Design review of the part built by this model. Coordinates are the model's own, in mm. A direction names the side the tool comes from. Give positions to 0.01 mm unless a question says otherwise; leave off trailing zeros. Order: outer loops, then holes, each group sorted by start corner. A loop starts at its lowest first (then second) coordinate and runs counter-clockwise, first axis right, second up. Notation, with made-up numbers: (54.5, 6) -> (85.5, 6) arc R17 ccw to (85.5, 19) -> close; hole circle Ø6 at (16, -30.75). An arc over 180 degrees is marked (long way). Return JSON: item names as keys, results as strings.
```python
from build123d import *

# Parameters (mm, degrees)
SKETCH1_W               = 80
SKETCH1_H               = 40
SKETCH1_R               = 2.25
BOSS_EXTRUDE1_DEPTH     = 5
BOSS_EXTRUDE1_2_DEPTH   = 5
SKETCH2_W               = 80
SKETCH2_H               = 5
BOSS_EXTRUDE2_DEPTH     = 71.3
SKETCH3_W               = 43.85
SKETCH3_H               = 62
BOSS_EXTRUDE3_DEPTH     = 5
SKETCH5_W               = 29.85
SKETCH5_H               = 38
CUT_EXTRUDE2_DEPTH      = 10
CUT_EXTRUDE1_REACH      = 114.097
SKETCH4_R               = 1.3
FILLET1_R               = 3
FILLET2_R               = 3
CUT_EXTRUDE3_DEPTH      = 133.735413511
CUT_EXTRUDE3_DEPTH_BACK = 133.735413511
SKETCH6_W               = 50
SKETCH6_H               = 38.3
FILLET3_R               = 3
SKETCH9_R               = 2.65
SKETCH9_R_2             = 1.05
BOSS_EXTRUDE5_DEPTH     = 4.75
SKETCH10_W              = 12
SKETCH10_H              = 6.8
CUT_EXTRUDE4_DEPTH      = 8


with BuildPart() as part:
    # Sketch1 → Boss-Extrude1 (new body)
    with BuildSketch(Plane(origin=(0, 0, 0), x_dir=(1, 0, 0), z_dir=(0, 1, 0))):
        with Locations((0, 46)):
            Rectangle(SKETCH1_W, SKETCH1_H)
        with Locations(Location((-30.625, 53.044055982, 0), (0, 0, 270))):
            Circle(SKETCH1_R, mode=Mode.SUBTRACT)
        with Locations(Location((30.625, 53.044055982, 0), (0, 0, 90))):
            Circle(SKETCH1_R, mode=Mode.SUBTRACT)
    extrude(amount=BOSS_EXTRUDE1_DEPTH)



with BuildPart() as body_2:
    # Sketch1 → Boss-Extrude1 2 (new body)
    with BuildSketch(Plane(origin=(0, 0, 0), x_dir=(1, 0, 0), z_dir=(0, 1, 0))):
        with Locations((0, -46)):
            Rectangle(SKETCH1_W, SKETCH1_H)
        with Locations(Location((30.625, -53.044055982, 0), (0, 0, 270))):
            Circle(SKETCH1_R, mode=Mode.SUBTRACT)
        with Locations(Location((-30.625, -53.044055982, 0), (0, 0, 90))):
            Circle(SKETCH1_R, mode=Mode.SUBTRACT)
    extrude(amount=BOSS_EXTRUDE1_2_DEPTH)


with BuildPart() as part_1:
    add(part.part)

    add(body_2.part)  # Boss-Extrude2 merges body 2
    # Sketch2 → Boss-Extrude2 (add)
    with BuildSketch(Plane(origin=(0, 5, 0), x_dir=(1, 0, 0), z_dir=(0, 1, 0))):
        with Locations((0, 28.5)):
            Rectangle(SKETCH2_W, SKETCH2_H)
        with Locations((0, -28.5)):
            Rectangle(SKETCH2_W, SKETCH2_H)
    extrude(amount=BOSS_EXTRUDE2_DEPTH)

    # Sketch3 → Boss-Extrude3 (add)
    with BuildSketch(Plane(origin=(0, 76.3, 0), x_dir=(1, 0, 0), z_dir=(0, 1, 0))):
        with Locations((-3.925, 0)):
            Rectangle(SKETCH3_W, SKETCH3_H)
    extrude(amount=BOSS_EXTRUDE3_DEPTH)

    # Sketch5 → Cut-Extrude2 (cut)
    with BuildSketch(Plane.XZ.offset(-76.3)):
        with Locations((-3.925, 0)):
            Rectangle(SKETCH5_W, SKETCH5_H)
    extrude(amount=-CUT_EXTRUDE2_DEPTH, mode=Mode.SUBTRACT)

    # Sketch4 → Cut-Extrude1 (cut, up to next)
    with BuildSketch(Plane(origin=(0, 81.3, 0), x_dir=(1, 0, 0), z_dir=(0, 1, 0)), mode=Mode.PRIVATE) as cut_extrude1_sk1:
        with Locations(Location((-23, 20, 0), (0, 0, 270))):
            Circle(SKETCH4_R)
    cut_extrude1_tool1 = extrude(cut_extrude1_sk1.sketch, amount=-CUT_EXTRUDE1_REACH, mode=Mode.PRIVATE) & part_1.part
    # Sketch4 → Cut-Extrude1 (cut, up to next)
    with BuildSketch(Plane(origin=(0, 81.3, 0), x_dir=(1, 0, 0), z_dir=(0, 1, 0)), mode=Mode.PRIVATE) as cut_extrude1_sk2:
        with Locations(Location((15, 20, 0), (0, 0, 270))):
            Circle(SKETCH4_R)
    cut_extrude1_tool2 = extrude(cut_extrude1_sk2.sketch, amount=-CUT_EXTRUDE1_REACH, mode=Mode.PRIVATE) & part_1.part
    # Sketch4 → Cut-Extrude1 (cut, up to next)
    with BuildSketch(Plane(origin=(0, 81.3, 0), x_dir=(1, 0, 0), z_dir=(0, 1, 0)), mode=Mode.PRIVATE) as cut_extrude1_sk3:
        with Locations(Location((15, -20, 0), (0, 0, 270))):
            Circle(SKETCH4_R)
    cut_extrude1_tool3 = extrude(cut_extrude1_sk3.sketch, amount=-CUT_EXTRUDE1_REACH, mode=Mode.PRIVATE) & part_1.part
    # Sketch4 → Cut-Extrude1 (cut, up to next)
    with BuildSketch(Plane(origin=(0, 81.3, 0), x_dir=(1, 0, 0), z_dir=(0, 1, 0)), mode=Mode.PRIVATE) as cut_extrude1_sk4:
        with Locations(Location((-23, -20, 0), (0, 0, 270))):
            Circle(SKETCH4_R)
    cut_extrude1_tool4 = extrude(cut_extrude1_sk4.sketch, amount=-CUT_EXTRUDE1_REACH, mode=Mode.PRIVATE) & part_1.part
    add(cut_extrude1_tool1.solids().sort_by_distance((-23, 81.3, -20))[0], mode=Mode.SUBTRACT)
    add(cut_extrude1_tool2.solids().sort_by_distance((15, 81.3, -20))[0], mode=Mode.SUBTRACT)
    add(cut_extrude1_tool3.solids().sort_by_distance((15, 81.3, 20))[0], mode=Mode.SUBTRACT)
    add(cut_extrude1_tool4.solids().sort_by_distance((-23, 81.3, 20))[0], mode=Mode.SUBTRACT)

    # Fillet1
    fillet1_edges = [part_1.edges().sort_by_distance(p)[0] for p in [
        (0, 5, -31),
        (-3.925, 76.3, -26),
        (-3.925, 76.3, 26),
        (0, 5, 31),
    ]]
    fillet(fillet1_edges, radius=FILLET1_R)

    # Fillet2
    fillet2_edges = [part_1.edges().sort_by_distance(p)[0] for p in [
        (18, 76.3, -28.5),
        (-25.85, 76.3, -28.5),
        (-25.85, 76.3, 28.5),
        (18, 76.3, 28.5),
    ]]
    fillet(fillet2_edges, radius=FILLET2_R)

    # Sketch6 → Cut-Extrude3 (cut, two sides: drawn at the far end of the back side and taken through both)
    with BuildSketch(Plane.XY.offset(31).offset(-CUT_EXTRUDE3_DEPTH_BACK)):
        with Locations((0, 42.15)):
            Rectangle(SKETCH6_W, SKETCH6_H)
    extrude(amount=CUT_EXTRUDE3_DEPTH + CUT_EXTRUDE3_DEPTH_BACK, mode=Mode.SUBTRACT)

    # Fillet3
    fillet3_edges = [part_1.edges().sort_by_distance(p)[0] for p in [
        (-25, 61.3, -28.5),
        (-25, 61.3, 28.5),
        (-25, 23, -28.5),
        (-25, 23, 28.5),
        (25, 23, -28.5),
        (25, 23, 28.5),
        (25, 61.3, -28.5),
        (25, 61.3, 28.5),
        (-18.85, 78.8, -19),
        (-18.85, 78.8, 19),
        (11, 78.8, 19),
        (11, 78.8, -19),
    ]]
    fillet(fillet3_edges, radius=FILLET3_R)

    # Sketch9 → Boss-Extrude5 (add)
    # profile 1 of 4: a face of its own
    with BuildSketch(Plane.XZ.offset(-76.3)):
        with Locations(Location((-23, 20, 0), (0, 0, 270))):
            Circle(SKETCH9_R)
        with Locations(Location((-23, 20, 0), (0, 0, 270))):
            Circle(SKETCH9_R_2, mode=Mode.SUBTRACT)
    # profile 2 of 4: a face of its own
    with BuildSketch(Plane.XZ.offset(-76.3)):
        with Locations(Location((-23, -20, 0), (0, 0, 270))):
            Circle(SKETCH9_R)
        with Locations(Location((-23, -20, 0), (0, 0, 270))):
            Circle(SKETCH9_R_2, mode=Mode.SUBTRACT)
    # profile 3 of 4: a face of its own
    with BuildSketch(Plane.XZ.offset(-76.3)):
        with Locations(Location((15, 20, 0), (0, 0, 270))):
            Circle(SKETCH9_R)
        with Locations(Location((15, 20, 0), (0, 0, 270))):
            Circle(SKETCH9_R_2, mode=Mode.SUBTRACT)
    # profile 4 of 4: a face of its own
    with BuildSketch(Plane.XZ.offset(-76.3)):
        with Locations(Location((15, -20, 0), (0, 0, 270))):
            Circle(SKETCH9_R)
        with Locations(Location((15, -20, 0), (0, 0, 270))):
            Circle(SKETCH9_R_2, mode=Mode.SUBTRACT)
    extrude(amount=BOSS_EXTRUDE5_DEPTH)

    # Sketch10 → Cut-Extrude4 (cut)
    with BuildSketch(Plane.XY.offset(31)):
        with Locations((6.7, 73.45)):
            Rectangle(SKETCH10_W, SKETCH10_H)
    extrude(amount=-CUT_EXTRUDE4_DEPTH, mode=Mode.SUBTRACT)


solid = part_1.part
```
Item 1: Mouldability with a two-part tool opening along X and no side actions: class faces 1 (the face through (18.86, 77.2, 28.46)), 2 (the face through (10.1, 78.83, 18.14)), 3 (the face through (-1, 5, 50)) as released by +X, released by -X, zero draft, split by the parting line, or undercut.
Result set:
{"face 1": "released by +X", "face 2": "undercut", "face 3": "zero draft"}
Item 2: Add section D-D (y = 24.5). Give the boundary of the cut face in (x, z).
Result set:
{"outline": "(-40, -31) -> (-24.6, -31) -> (-24.6, -26) -> (-40, -26) -> close; (-40, 26) -> (-24.6, 26) -> (-24.6, 31) -> (-40, 31) -> close; (24.6, -31) -> (40, -31) -> (40, -26) -> (24.6, -26) -> close; (24.6, 26) -> (40, 26) -> (40, 31) -> (24.6, 31) -> close"}
Item 3: Wall thickness on L1, parallel to X at y = 79.05, z = -20; L2, parallel to Z at x = -3.5, y = 71; L3, parallel to Y at x = -15.5, z = 30.5: over which ranges is each line inside the solid? List them lowest first. Write a range as [from, to].
Result set:
{"L1": "x = [-25.85, -24.3], [-21.7, 13.7], [16.3, 18]", "L2": "z = [-31, -26], [26, 31]", "L3": "y = [0, 23], [61.3, 81.3]"}
Item 4: Machinability: for faces 4 (the face through (-4, 79, -19)), 5 (the face through (0, 61.3, 28)), 6 (the face through (-1, 5, -50)), 7 (the face through (7, 70.05, 29)), 8 (the face through (-24, 71.55, 19)), which of the approach directions +Z, -Z, +X, -X, +Y, -Y give a long, thin tool a straight path to every point of the face, cutting with its end or side? Answer none if there is none.
Result set:
{"face 4": "+Y, -Y", "face 5": "+Z, -Z", "face 6": "-Z, +X, -X, +Y", "face 7": "+Z", "face 8": "+X, -X, -Y"}
Item 5: Add section A-A (x = 2.5). Give the number of separate pieces and of enclosed holes in the cut face, plus the area to 3 significant figures.
Result set:
{"separate pieces": "5", "enclosed holes": "0", "area": "820 mm^2"}
Item 6: Add section C-C (y = 35). Give the boundary of the cut face in (x, z), plus the area to 3 significant figures.
Result set:
{"outline": "(-40, -31) -> (-25, -31) -> (-25, -26) -> (-40, -26) -> close; (-40, 26) -> (-25, 26) -> (-25, 31) -> (-40, 31) -> close; (25, -31) -> (40, -31) -> (40, -26) -> (25, -26) -> close; (25, 26) -> (40, 26) -> (40, 31) -> (25, 31) -> close", "area": "300 mm^2"}
Item 7: For pin 1 (1.3 mm diameter, centred on x = -23.5, z = -20, fed in from +Y); pin 2 (2.5 mm diameter, centred on x = 5, z = 27.5, fed in from -Y); pin 3 (3 mm diameter, centred on x = -23, z = 20, fed in from -Y); pin 4 (6.5 mm diameter, centred on y = 76.5, z = 13.5, fed in from +X), all flat-tipped, find the tip position at first contact; note any pin that passes through.
Result set:
{"pin 1": "stops at y = 76.3", "pin 2": "stops at y = 0", "pin 3": "stops at y = 71.55", "pin 4": "stops at x = 18"}
Item 8: Add section B-B (z = -5). Give the boundary of the cut face in (x, y), plus the area to 3 significant figures.
Result set:
{"outline": "(-25.85, 76.3) -> (-18.85, 76.3) -> (-18.85, 81.3) -> (-25.85, 81.3) -> close; (11, 76.3) -> (18, 76.3) -> (18, 81.3) -> (11, 81.3) -> close", "area": "70.0 mm^2"}
